Can you work these out from the drawing? Everything is in mm from the part's minimum corner. A direction names the side the tool comes from. Give positions to 0.01 mm unless a question says otherwise; leave off trailing zeros. Write each loop counter-clockwise with the first axis right and the second up, starting at its lowest first coordinate (ties: lowest second). Pieces come first, ordered by that corner, then holes. Notation, with made-up numbers: (64.5, 58.25) - (75.5, 58.25) arc R15 ccw to (75.5, 72.25) - close; hole circle Ø6 at (-16, -32.75). An arc over 180 degrees is marked (long way). Return JSON: item names as keys, results as strings. Group by question number.
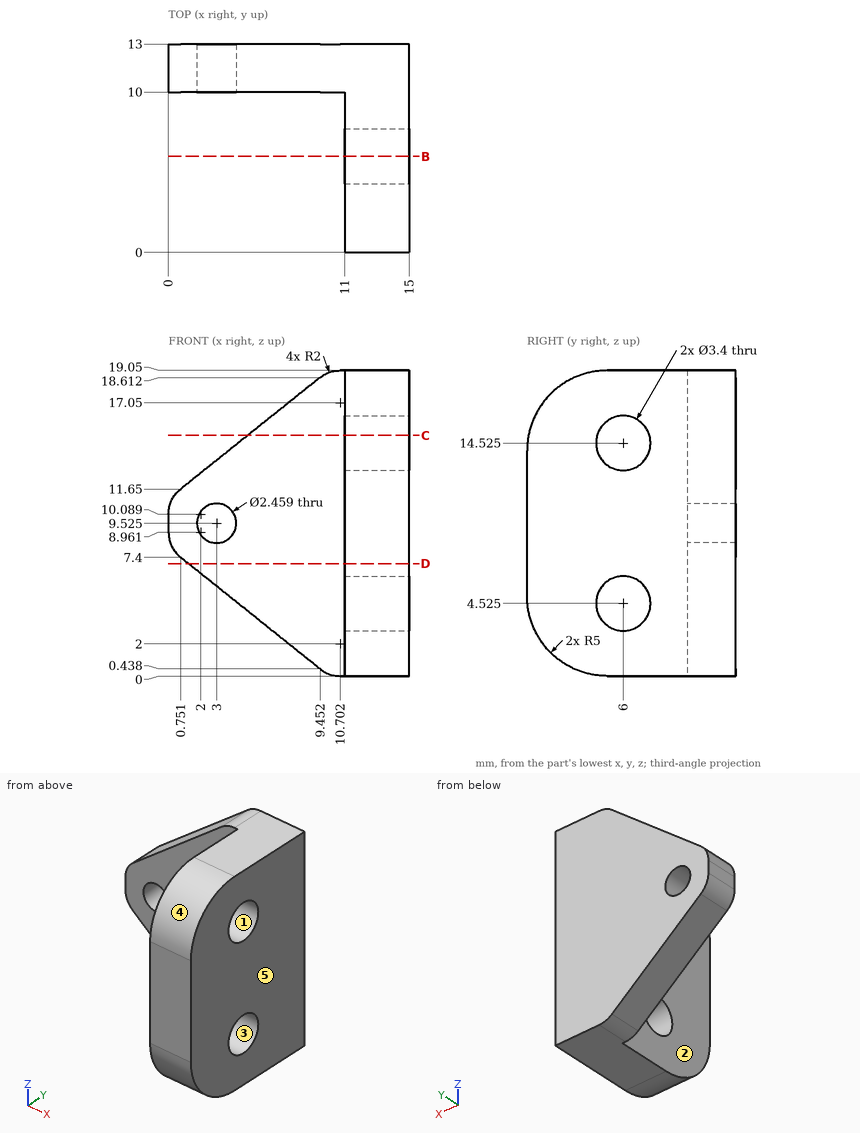
1) On a 3-axis mill with a long thin cutter (end or side, diameter ignored), from which of +Z, -Z, +X, -X, +Y, -Y can I reach the whole of each face in a straight line? I mean the marked faces 1 and 2. Say none if no direction works.
2) Will these pins go through, and if not, where does the flat tip stop? pin 1 Ø6 at (y, z) = (6.5, 8.5) entering from -X; pin 2 Ø2.5 at (y, z) = (6, 14.525) entering from +X; pin 3 Ø5 at (x, y) = (5.5, 9) entering from +Z; pin 4 Ø3.5 at (x, z) = (4, 14) entering from -Y.
3) Imagine slicing it at B-B, the plane y = 6. Count the separate pieces of the cut face and the enclosed holes in it, and give its area (3 significant figures).
4) We'd pull the mould along Z, two halves only. Please class the marked faces 3, 4 and 5: pulls with the +Z half, pulls with the -Z half, needs draft (parallel to the pull), parting line crosses it, or undercut.
5) I need wall thicknesses on line 1 along X through (y, z) = (5.5, 12.5); line 2 along Y through (x, z) = (10.75, 9.25); line 3 along Y through (x, z) = (11.25, 4). Which ranges of each line are inside material? Lowest first, please.
6) Imagine slicing it at C-C, the plane z = 15. Write out the boundary of the cut face in (x, y).
7) Imagine slicing it at D-D, the plane z = 7. Write out the boundary of the cut face in (x, y).
Resolved:
{
 "1": {"face 1": "+X, -X", "face 2": "+Z, -Z, -X, -Y"},
 "2": {"pin 1": "x = 11", "pin 2": "through", "pin 3": "z = 17.28", "pin 4": "y = 10"},
 "3": {"separate pieces": "3", "enclosed holes": "0", "area": "49.0 mm^2"},
 "4": {"face 3": "undercut", "face 4": "pulls with the +Z half", "face 5": "needs draft"},
 "5": {"line 1": "11 to 15", "line 2": "10 to 13", "line 3": "0.1 to 4.38, 7.62 to 13"},
 "6": {"outline": "(4.94, 10) - (11, 10) - (11, 7.63) - (15, 7.63) - (15, 13) - (4.94, 13) - close; (11, 0.09) - (15, 0.09) - (15, 4.37) - (11, 4.37) - close"},
 "7": {"outline": "(1.25, 10) - (11, 10) - (11, 0) - (15, 0) - (15, 13) - (1.25, 13) - close"}
}
